```python
from build123d import *

# Parameters (mm, degrees)
SKETCH1_W               = 63.5
SKETCH1_H               = 57.15
BOSS_EXTRUDE5_DEPTH     = 148.59
SKETCH5_OUTSIDE_W       = 99.78
SKETCH5_OUTSIDE_H       = 93.43
SKETCH5_OUTSIDE_W_2     = 63.5
SKETCH5_OUTSIDE_H_2     = 57.15
SKETCH5_OUTSIDE_R       = 25.4
CUT_EXTRUDE4_DEPTH      = 146.05
SKETCH8_W               = 63.5
SKETCH8_H               = 57.15
SKETCH8_R               = 12.740402439
BOSS_EXTRUDE6_DEPTH     = 2.54
CUT_EXTRUDE5_REACH      = 175.605
CUT_EXTRUDE5_END_RADIUS = 25.4
SKETCH9_R               = 10.16
CUT_EXTRUDE6_REACH      = 175.605
CUT_EXTRUDE6_END_RADIUS = 25.4
SKETCH10_R              = 10.16


with BuildPart() as part:
    # Sketch1 → Boss-Extrude5 (new body)
    with BuildSketch(Plane.XY):
        with Locations((31.75, 28.575)):
            Rectangle(SKETCH1_W, SKETCH1_H)
    extrude(amount=BOSS_EXTRUDE5_DEPTH)

    # Sketch5 outside → Cut-Extrude4 (cut)
    # profile 1 of 2: a face of its own
    with BuildSketch(Plane.XY.offset(148.59)):
        with Locations((31.75, 28.575)):
            Rectangle(SKETCH5_OUTSIDE_W, SKETCH5_OUTSIDE_H)
        with Locations((31.75, 28.575)):
            Rectangle(SKETCH5_OUTSIDE_W_2, SKETCH5_OUTSIDE_H_2, mode=Mode.SUBTRACT)
    # profile 2 of 2: a face of its own
    with BuildSketch(Plane.XY.offset(148.59)):
        with Locations((31.75, 28.575)):
            Circle(SKETCH5_OUTSIDE_R)
    extrude(amount=-CUT_EXTRUDE4_DEPTH, mode=Mode.SUBTRACT)

    # Sketch8 → Boss-Extrude6 (add, symmetric)
    with BuildSketch(Plane.XY.offset(148.59)):
        with Locations((31.75, 28.575)):
            Rectangle(SKETCH8_W, SKETCH8_H)
        with Locations((31.75, 28.575)):
            Circle(SKETCH8_R, mode=Mode.SUBTRACT)
    extrude(amount=BOSS_EXTRUDE6_DEPTH, both=True)

    # Cut-Extrude5: up to this cylinder (the profile starts outside it)
    cut_extrude5_end = Plane(origin=(31.75, 28.575, 71.628), z_dir=(0, 0, 1)) * Cylinder(CUT_EXTRUDE5_END_RADIUS, 403.01, mode=Mode.PRIVATE)
    # Sketch9 → Cut-Extrude5 (cut, up to the surface)
    with BuildSketch(Plane(origin=(0, 57.15, 0), x_dir=(1, 0, 0), z_dir=(0, 1, 0)), mode=Mode.PRIVATE) as cut_extrude5_sk1:
        with Locations(Location((31.75, -71.628, 0), (0, 0, 270))):
            Circle(SKETCH9_R)
    cut_extrude5_tool1 = extrude(cut_extrude5_sk1.sketch, amount=-CUT_EXTRUDE5_REACH, mode=Mode.PRIVATE) - cut_extrude5_end
    add(cut_extrude5_tool1.solids().sort_by_distance((31.75, 57.15, 71.628))[0], mode=Mode.SUBTRACT)

    # Cut-Extrude6: up to this cylinder (the profile starts outside it)
    cut_extrude6_end = Plane(origin=(31.75, 28.575, 88.265), z_dir=(0, 0, 1)) * Cylinder(CUT_EXTRUDE6_END_RADIUS, 477.94, mode=Mode.PRIVATE)
    # Sketch10 → Cut-Extrude6 (cut, up to the surface)
    with BuildSketch(Plane.XZ, mode=Mode.PRIVATE) as cut_extrude6_sk1:
        with Locations(Location((17.78, 81.534, 0), (0, 0, 270))):
            Circle(SKETCH10_R)
    cut_extrude6_tool1 = extrude(cut_extrude6_sk1.sketch, amount=-CUT_EXTRUDE6_REACH, mode=Mode.PRIVATE) - cut_extrude6_end
    add(cut_extrude6_tool1.solids().sort_by_distance((17.78, 0, 81.534))[0], mode=Mode.SUBTRACT)
    # Sketch10 → Cut-Extrude6 (cut, up to the surface)
    with BuildSketch(Plane.XZ, mode=Mode.PRIVATE) as cut_extrude6_sk2:
        with Locations(Location((44.45, 125.73, 0), (0, 0, 270))):
            Circle(SKETCH10_R)
    cut_extrude6_tool2 = extrude(cut_extrude6_sk2.sketch, amount=-CUT_EXTRUDE6_REACH, mode=Mode.PRIVATE) - cut_extrude6_end
    add(cut_extrude6_tool2.solids().sort_by_distance((44.45, 0, 125.73))[0], mode=Mode.SUBTRACT)
    # Sketch10 → Cut-Extrude6 (cut, up to the surface)
    with BuildSketch(Plane.XZ, mode=Mode.PRIVATE) as cut_extrude6_sk3:
        with Locations(Location((44.45, 50.8, 0), (0, 0, 270))):
            Circle(SKETCH10_R)
    cut_extrude6_tool3 = extrude(cut_extrude6_sk3.sketch, amount=-CUT_EXTRUDE6_REACH, mode=Mode.PRIVATE) - cut_extrude6_end
    add(cut_extrude6_tool3.solids().sort_by_distance((44.45, 0, 50.8))[0], mode=Mode.SUBTRACT)


solid = part.part
```
The model under review builds one solid part; all positions refer to its coordinate system, in mm. A direction names the side the tool comes from. Round coordinates to 2 decimals unless told otherwise and drop trailing zeros. Write each loop counter-clockwise with the first axis right and the second up, starting at its lowest first coordinate (ties: lowest second). Pieces come first, ordered by that corner, then holes. Notation, with made-up numbers: (15.5, 87.25) - (20.5, 87.25) arc R24 cw to (20.5, 116.25) - close; hole circle Ø8 at (-37, 47). An arc over 180 degrees is marked (long way). One line per question, with ' | ' between items.
Item 1: Add section B-B, the plane z = 50.8. Give the boundary of the cut face in (x, y) (3 decimals).
Resolved:
outline: (0, 0) - (34.29, 0) - (34.29, 3.302) arc R25.4 cw (long way) to (54.61, 17.503) - (54.61, 0) - (63.5, 0) - (63.5, 57.15) - (0, 57.15) - close
Item 2: The part is to be moulded in two halves that separate along Y. For faces 4 (the face through (17, 57.15, 75)), 5 (the face through (20, 23, 146.05)), 6 (the face through (0, 28, 75)), say which applies: pulls with the +Y half, pulls with the -Y half, needs draft (parallel to the pull), parting line crosses it, or undercut.
Resolved:
face 4: pulls with the +Y half | face 5: undercut | face 6: needs draft
Item 3: To check wall thickness, follow probe 1 along Z at (x, y) = (51.5, 39.5); probe 2 along Y at (x, z) = (32.5, 22); probe 3 along Y at (x, z) = (20, 47). State the ranges of each line that lie inside material, in increasing order.
Resolved:
probe 1: z = 0 to 2.54, 146.05 to 151.13 | probe 2: y = 0 to 3.19, 53.96 to 57.15 | probe 3: y = 0 to 6.06, 51.09 to 57.15
Item 4: Add section D-D, the plane z = 100.5. Give the boundary of the cut face in (x, y) (3 decimals).
Resolved:
outline: (0, 0) - (63.5, 0) - (63.5, 57.15) - (0, 57.15) - close; hole circle Ø50.8 at (31.75, 28.575)
Item 5: For P1, Ø1.5, axis at x = 40, y = 33.5, coming from the +Z side; P2, Ø3, axis at x = 46.5, z = 64.5, coming from the -Y side; P3, Ø18.5, axis at x = 31.75, z = 71.628, coming from the +Y side, all flat-tipped, find the tip position at first contact; note any pin that passes through.
Resolved:
P1: stops at z = 2.54 | P2: stops at y = 0 | P3: stops at y = 4.92
Item 6: Add section A-A, the plane x = 31.75. Give the boundary of the cut face in (y, z) (3 decimals).
Resolved:
outline: (0, 0) - (57.15, 0) - (57.15, 61.468) - (53.975, 61.468) - (53.975, 2.54) - (3.175, 2.54) - (3.175, 146.05) - (15.835, 146.05) - (15.835, 151.13) - (0, 151.13) - close; (41.315, 146.05) - (53.975, 146.05) - (53.975, 81.788) - (57.15, 81.788) - (57.15, 151.13) - (41.315, 151.13) - close
Item 7: Add section C-C, the plane y = 10.5. Give the boundary of the cut face in (x, z), then the cut area to 3 significant figures.
Resolved:
outline: (0, 0) - (63.5, 0) - (63.5, 151.13) - (0, 151.13) - close; hole (13.9, 2.54) - (49.6, 2.54) - (49.6, 42.04) arc R10.16 ccw to (49.6, 59.56) - (49.6, 116.97) arc R10.16 ccw to (49.6, 134.49) - (49.6, 146.05) - (13.9, 146.05) - (13.9, 90.93) arc R10.16 ccw to (13.9, 72.14) - close | area: 4,260 mm2
Item 8: For faces 1 (the face through (43.902, 32.402, 148.554)), 2 (the face through (13.03, 45.74, 75.3)), 3 (the face through (54.524, 4.74, 52.123)), list the 3-axis set-ups (+Z, -Z, +X, -X, +Y, -Y) from which the entire face can be reached by the end or side of a thin tool; tool diameter is ignored.
Resolved:
face 1: +Z | face 2: none | face 3: -Y
